Here's the drawing with two shaded views (mm, measured from the low corner). I have some questions. Coordinates: 2 decimals unless noted, no trailing zeros. Write each loop counter-clockwise with the first axis right and the second up, starting at its lowest first coordinate (ties: lowest second). Pieces come first, ordered by that corner, then holes.
Item 1: If we section it at B-B (z = 7.5): Please give me the cut outline in (x, y) (1 decimal).
Item 2: If we section it at C-C (y = 3.5): Count the separate pieces of the cut face and the enclosed holes in it, then the cut area to 3 significant figures.
Item 3: If we section it at A-A (z = 20.32): Please give me the cut outline in (x, y) (1 decimal).
Item 4: If we section it at D-D (x = 17.5): Please give me the cut outline in (y, z) (1 decimal).
Item 5: I'm going to push flat-ended pins straight in: pin 1 Ø2 at (y, z) = (3.5, 16.5) entering from -X; pin 2 Ø4.5 at (x, z) = (16.32, 20.32) entering from -Y. Where does each tip first touch, or does it pass through?
Item 6: If I drill on line 1 (X direction, y = 2.25, z = 20); line 2 (X direction, y = 1, z = 18.5) (1 decimal); line 3 (Z direction, x = 13.5, y = 3) (1 decimal), over which ranges is the centre line in solid material (lowest first)?
Item 7: We'd pull the mould along X, two halves only. Please class the marked faces 1, 2 and 3: +X half, -X half, draft (parallel to the pull), parting line (faces both ways), or undercut.
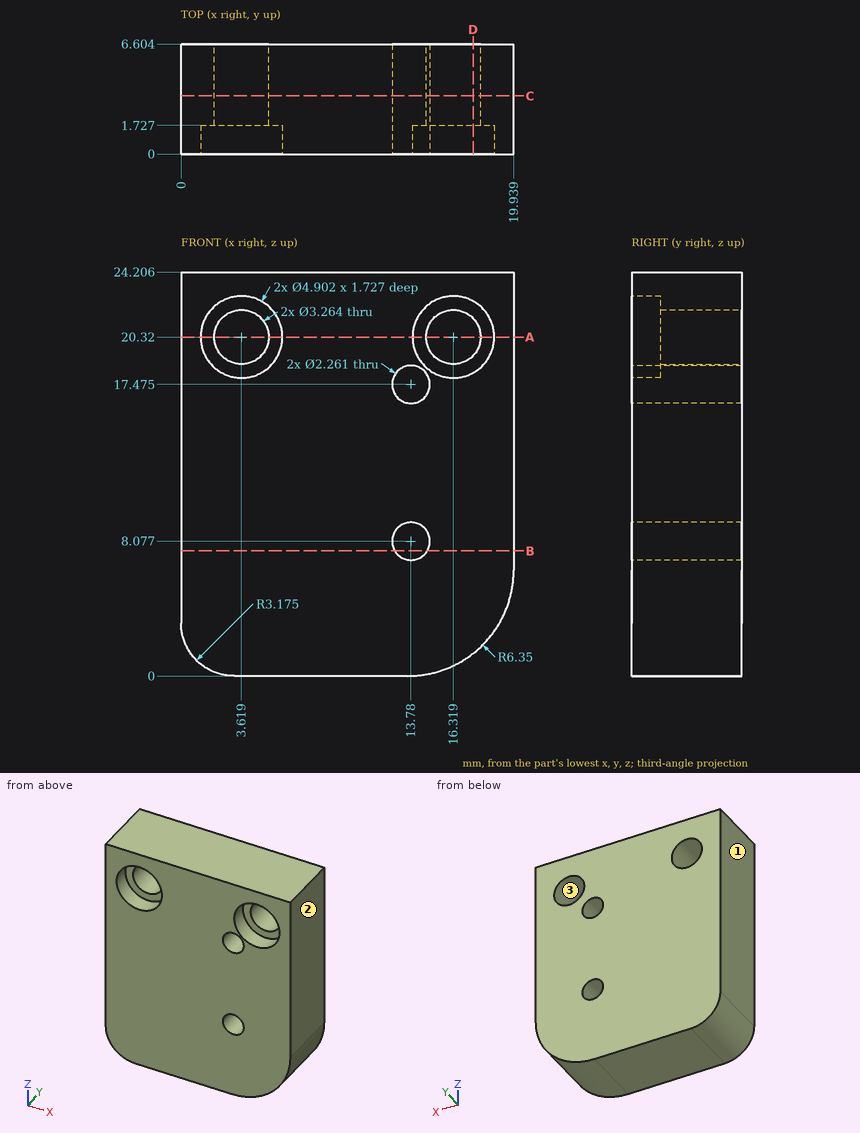
Answer list:
1. outline: (0, 0) - (12.8, 0) - (12.8, 6.6) - (0, 6.6) - close; (14.8, 0) - (19.9, 0) - (19.9, 6.6) - (14.8, 6.6) - close
2. separate pieces: 1
2. enclosed holes: 4
2. area: 447 mm2
3. outline: (0, 0) - (1.2, 0) - (1.2, 1.7) - (2, 1.7) - (2, 6.6) - (0, 6.6) - close; (5.3, 1.7) - (6.1, 1.7) - (6.1, 0) - (13.9, 0) - (13.9, 1.7) - (14.7, 1.7) - (14.7, 6.6) - (5.3, 6.6) - close; (18, 1.7) - (18.8, 1.7) - (18.8, 0) - (19.9, 0) - (19.9, 6.6) - (18, 6.6) - close
4. outline: (0, 1.3) - (6.6, 1.3) - (6.6, 19.2) - (1.7, 19.2) - (1.7, 18.2) - (0, 18.2) - close; (0, 22.5) - (1.7, 22.5) - (1.7, 21.4) - (6.6, 21.4) - (6.6, 24.2) - (0, 24.2) - close
5. pin 1: stops at x = 0
5. pin 2: stops at y = 1.73
6. line 1: x = 0 to 2.02, 5.22 to 14.72, 17.92 to 19.94
6. line 2: x = 0 to 2, 5.3 to 13.3, 14.3 to 14.7, 18 to 19.9
6. line 3: z = 0 to 7, 9.2 to 16.4, 18.6 to 24.2
7. face 1: -X half
7. face 2: +X half
7. face 3: undercut
